Autodesk Fusion 360 part; units mm, degrees
sketch "Sketch1" plane through (0, 0, 0) normal (0, 0, 1) x (1, 0, 0)
  arc A0 (21.59, 0) -> (24.13, 2.54) centre (21.59, 2.54) ccw
  arc A1 (0, 2.54) -> (2.54, 0) centre (2.54, 2.54) ccw
  line L0 (21.59, 0) -> (2.54, 0)
  arc A2 (2.54, 15.24) -> (0, 12.7) centre (2.54, 12.7) ccw
  line L1 (24.13, 12.7) -> (24.13, 2.54)
  line L2 (0, 2.54) -> (0, 12.7)
  line L3 (2.54, 15.24) -> (21.59, 15.24)
  arc A3 (24.13, 12.7) -> (21.59, 15.24) centre (21.59, 12.7) ccw
  arc A4 (20.9931, 9.293) -> (19.9009, 9.293) centre (20.447, 9.293) ccw
  line L4 (2.159, 1.651) -> (3.937, 1.651)
  line L5 (3.937, 1.651) -> (3.937, 3.429)
  line L6 (2.159, 1.651) -> (3.937, 1.651)
  line L7 (3.937, 1.651) -> (3.937, 3.429)
  line L8 (3.937, 3.429) -> (2.159, 3.429)
  arc A5 (20.9931, 5.793) -> (19.9009, 5.793) centre (20.447, 5.793) ccw
  arc A6 (19.9009, 9.293) -> (20.9931, 9.293) centre (20.447, 9.293) ccw
  arc A7 (19.9009, 9.293) -> (20.9931, 9.293) centre (20.447, 9.293) ccw
  line L9 (2.159, 3.429) -> (2.159, 1.651)
  line L10 (2.159, 3.429) -> (2.159, 1.651)
  arc A8 (20.9931, 9.293) -> (19.9009, 9.293) centre (20.447, 9.293) ccw
  arc A9 (19.9009, 5.793) -> (20.9931, 5.793) centre (20.447, 5.793) ccw
  arc A10 (20.9931, 5.793) -> (19.9009, 5.793) centre (20.447, 5.793) ccw
  line L11 (3.937, 3.429) -> (2.159, 3.429)
  arc A11 (19.9009, 5.793) -> (20.9931, 5.793) centre (20.447, 5.793) ccw
  circle A12 centre (21.59, 2.286) radius 1.27
  circle A13 centre (21.59, 12.954) radius 1.27
  circle A14 centre (3.048, 2.54) radius 0.635
  circle A15 centre (3.048, 5.08) radius 0.635
  circle A16 centre (3.048, 7.62) radius 0.635
  circle A17 centre (3.048, 10.16) radius 0.635
  circle A18 centre (3.048, 12.7) radius 0.635
  circle A19 centre (3.048, 5.08) radius 1
  circle A20 centre (3.048, 7.62) radius 1
  circle A21 centre (3.048, 10.16) radius 1
  circle A22 centre (3.048, 12.7) radius 1
  dimension "d1" = 2.54
  dimension "d2" = 2.54
  dimension "d5" = 1.27
  dimension "d8" = 0
  dimension "d9" = 2.54
  dimension "d10" = 2
  dimension "d13" = 0
  dimension "d14" = 2.54
extrude "Extrude1" add sketch "Sketch1" along normal blind 1.6 contours A0 A1 L0 A2 L1 L2 L3 A3 | L4 L5 L6 L7 L8 L9 L10 L11 | A19 | A20 | A21 | A22
extrude "Extrude2" add sketch "Sketch1" along normal blind 0.2 from surface at 1.6 contours L4 L5 L6 L7 L8 L9 L10 L11 | A19 | A20 | A21 | A22
sketch "Sketch2" plane through (0, 0, 1.6) normal (0, 0, 1) x (-1, 0, 0)
  circle A0 centre (-3.048, -12.7) radius 1
  line L0 (-3.937, -1.651) -> (-2.159, -1.651)
  line L1 (-2.159, -1.651) -> (-2.159, -3.429)
  line L2 (-2.159, -3.429) -> (-3.937, -3.429)
  line L3 (-3.937, -3.429) -> (-3.937, -1.651)
  circle A1 centre (-3.048, -10.16) radius 1
  circle A2 centre (-3.048, -5.08) radius 1
  circle A3 centre (-3.048, -7.62) radius 1
  circle A4 centre (-21.59, -2.286) radius 1.27
  circle A5 centre (-20.447, -9.293) radius 0.5461
  circle A6 centre (-21.59, -12.954) radius 1.27
  circle A7 centre (-20.447, -5.793) radius 0.5461
  arc A8 (-21.59, 0) -> (-24.13, -2.54) centre (-21.59, -2.54) ccw
  line L4 (-24.13, -2.54) -> (-24.13, -12.7)
  arc A9 (-24.13, -12.7) -> (-21.59, -15.24) centre (-21.59, -12.7) ccw
  line L5 (-21.59, -15.24) -> (-2.54, -15.24)
  arc A10 (-2.54, -15.24) -> (0, -12.7) centre (-2.54, -12.7) ccw
  line L6 (0, -12.7) -> (0, -2.54)
  arc A11 (0, -2.54) -> (-2.54, 0) centre (-2.54, -2.54) ccw
  line L7 (-2.54, 0) -> (-21.59, 0)
  line L8 (-7.25, -3.5) -> (-5.75, -3.5)
  line L9 (-5.75, -3.5) -> (-5.75, -6.5)
  line L10 (-5.75, -6.5) -> (-7.25, -6.5)
  line L11 (-7.25, -6.5) -> (-7.25, -3.5)
  line L12 (-7.25, -3.5) -> (-5.75, -6.5) construction
  line L13 (-5.75, -3.5) -> (-7.25, -6.5) construction
  line L14 (-9.75, -2.5) -> (-8.25, -2.5)
  line L15 (-8.25, -2.5) -> (-8.25, -5.5)
  line L16 (-8.25, -5.5) -> (-9.75, -5.5)
  line L17 (-9.75, -5.5) -> (-9.75, -2.5)
  line L18 (-9.75, -2.5) -> (-8.25, -5.5) construction
  line L19 (-8.25, -2.5) -> (-9.75, -5.5) construction
  line L20 (-15, -3.5) -> (-11, -3.5)
  line L21 (-11, -3.5) -> (-11, -7.5)
  line L22 (-11, -7.5) -> (-15, -7.5)
  line L23 (-15, -7.5) -> (-15, -3.5)
  line L24 (-15, -3.5) -> (-11, -7.5) construction
  line L25 (-11, -3.5) -> (-15, -7.5) construction
  line L26 (-9, -9.25) -> (-6, -9.25)
  line L27 (-6, -9.25) -> (-6, -10.75)
  line L28 (-6, -10.75) -> (-9, -10.75)
  line L29 (-9, -10.75) -> (-9, -9.25)
  line L30 (-9, -9.25) -> (-6, -10.75) construction
  line L31 (-6, -9.25) -> (-9, -10.75) construction
  line L32 (-6.5, -7.25) -> (-9.5, -7.25)
  line L33 (-9.5, -7.25) -> (-9.5, -8.75)
  line L34 (-9.5, -8.75) -> (-6.5, -8.75)
  line L35 (-6.5, -8.75) -> (-6.5, -7.25)
  line L36 (-6.5, -7.25) -> (-9.5, -8.75) construction
  line L37 (-9.5, -7.25) -> (-6.5, -8.75) construction
  circle A12 centre (-8, -13) radius 1.25
  line L38 (-14, -12) -> (-11, -12)
  line L39 (-11, -12) -> (-11, -13.5)
  line L40 (-11, -13.5) -> (-14, -13.5)
  line L41 (-14, -13.5) -> (-14, -12)
  line L42 (-14, -12) -> (-11, -13.5) construction
  line L43 (-11, -12) -> (-14, -13.5) construction
  line L44 (-12, -8.5) -> (-10.5, -8.5)
  line L45 (-10.5, -8.5) -> (-10.5, -11.5)
  line L46 (-10.5, -11.5) -> (-12, -11.5)
  line L47 (-12, -11.5) -> (-12, -8.5)
  line L48 (-12, -8.5) -> (-10.5, -11.5) construction
  line L49 (-10.5, -8.5) -> (-12, -11.5) construction
  line L50 (-19, -2.5) -> (-16, -2.5)
  line L51 (-16, -2.5) -> (-16, -4)
  line L52 (-16, -4) -> (-19, -4)
  line L53 (-19, -4) -> (-19, -2.5)
  line L54 (-19, -2.5) -> (-16, -4) construction
  line L55 (-16, -2.5) -> (-19, -4) construction
  line L56 (-19, -6) -> (-19, -4.5)
  line L57 (-19, -4.5) -> (-16, -4.5)
  line L58 (-16, -4.5) -> (-16, -6)
  line L59 (-16, -6) -> (-19, -6)
  line L60 (-19, -8) -> (-19, -6.5)
  line L61 (-19, -6.5) -> (-16, -6.5)
  line L62 (-16, -6.5) -> (-16, -8)
  line L63 (-16, -8) -> (-19, -8)
  line L64 (-19, -10) -> (-19, -8.5)
  line L65 (-19, -8.5) -> (-16, -8.5)
  line L66 (-16, -8.5) -> (-16, -10)
  line L67 (-16, -10) -> (-19, -10)
  line L68 (-6.5, -11.5) -> (-9.5, -11.5)
  line L69 (-9.5, -11.5) -> (-9.5, -14.5)
  line L70 (-9.5, -14.5) -> (-6.5, -14.5)
  line L71 (-6.5, -14.5) -> (-6.5, -11.5)
  line L72 (-6.5, -11.5) -> (-9.5, -14.5) construction
  line L73 (-9.5, -11.5) -> (-6.5, -14.5) construction
  point P0 (-6.5, -5)
  point P1 (-9, -4)
  point P2 (-13, -5.5)
  point P3 (-7.5, -10)
  point P4 (-8, -8)
  point P5 (-12.5, -12.75)
  point P6 (-11.25, -10)
  point P7 (-17.5, -3.25)
  point P8 (-8, -13)
  dimension "d18" = 1.5
  dimension "d19" = 3
  dimension "d20" = 1.5
  dimension "d21" = 3
  dimension "d22" = 4
  dimension "d23" = 4
  dimension "d24" = 3
  dimension "d25" = 1.5
  dimension "d26" = 3
  dimension "d27" = 1.5
  dimension "d28" = 2.5
  dimension "d29" = 1.5
  dimension "d30" = 3
  dimension "d31" = 3
  dimension "d32" = 1.5
  dimension "d33" = 3
  dimension "d34" = 1.5
  dimension "d37" = 0
  dimension "d38" = -2
  dimension "d43" = 3
  dimension "d44" = 3
extrude "Extrude3" add sketch "Sketch2" along normal blind 0.5 contours L8 L9 L10 L11 | L32 L33 L34 L35 | L44 L45 L46 L47
extrude "Extrude4" add sketch "Sketch2" along normal blind 1 contours L14 L15 L16 L17 | L20 L21 L22 L23 | L26 L27 L28 L29 | L38 L39 L40 L41 | L50 L51 L52 L53 | L56 L57 L58 L59 | L60 L61 L62 L63 | L64 L65 L66 L67
extrude "Extrude5" add sketch "Sketch2" along normal blind 1 contours A12 | L68 L69 L70 L71
extrude "Extrude6" add sketch "Sketch2" along normal blind 0.5 from surface at 1 contours A12
Input: part model. Units: mm. Frame: model coordinates. A direction names the side the tool comes from. Give positions to 0.01 mm unless a question says otherwise; leave off trailing zeros. Order: outer loops, then holes, each group sorted by start corner. A loop starts at its lowest first (then second) coordinate and runs counter-clockwise, first axis right, second up. Notation, with made-up numbers: (25.5, -8) - (52.5, -8) arc R26 cw to (52.5, 18) - close; hole circle Ø9 at (-18.75, 45.25). An arc over 180 degrees is marked (long way). Use a Markdown table: item, result.
(1) Section query B-B (x = 8). Output: boundary loops of the cut face in (y, z), then the cut area to 3 significant figures.
Computed values:
| item | result |
|---|---|
| outline | (0, 0) - (15.24, 0) - (15.24, 1.6) - (14.5, 1.6) - (14.5, 2.6) - (14.25, 2.6) - (14.25, 3.1) - (11.75, 3.1) - (11.75, 2.6) - (11.5, 2.6) - (11.5, 1.6) - (10.75, 1.6) - (10.75, 2.6) - (9.25, 2.6) - (9.25, 1.6) - (8.75, 1.6) - (8.75, 2.1) - (7.25, 2.1) - (7.25, 1.6) - (0, 1.6) - close |
| area | 30.9 mm2 |
(2) Section query A-A (y = 10.5). Output: boundary loops of the cut face in (x, z), then the cut area to 3 significant figures.
Computed values:
| item | result |
|---|---|
| outline | (0, 0) - (2.51, 0) - (2.51, 1.8) - (2.11, 1.8) - (2.11, 1.6) - (0, 1.6) - close; (3.58, 0) - (24.13, 0) - (24.13, 1.6) - (12, 1.6) - (12, 2.1) - (10.5, 2.1) - (10.5, 1.6) - (9, 1.6) - (9, 2.6) - (6, 2.6) - (6, 1.6) - (3.99, 1.6) - (3.99, 1.8) - (3.58, 1.8) - close |
| area | 40.8 mm2 |
(3) Access query for faces 1 (the flat face through (16, 7, 2)), 2 (the flat face through (17, 10, 2)), 3 (the flat face through (8, 11.5, 2)), 4 (the flat face through (13, 7.5, 2)). Directions: +Z, -Z, +X, -X, +Y, -Y. A direction counts if a zero-diameter tool reaches every point of the face in a straight line with its end or side. Return the directions, or none.
Computed values:
| item | result |
|---|---|
| face 1 | +Z, +Y, -Y |
| face 2 | +Z, +X, +Y |
| face 3 | +Z, -X |
| face 4 | +Z |
(4) Pin query (flat end, axial travel): pin 1 (0.5 mm diameter, centred on y = 9, z = 2, fed in from +X); pin 2 (1.6 mm diameter, centred on x = 7, y = 5, fed in from +Z); pin 3 (2 mm diameter, centred on x = 21.59, y = 2.286, fed in from +Z); pin 4 (0.5 mm diameter, centred on x = 17.5, z = 2, fed in from +Y). Return the tip coordinate at first contact, or that it passes through.
Computed values:
| item | result |
|---|---|
| pin 1 | stops at x = 19 |
| pin 2 | stops at z = 2.1 |
| pin 3 | passes through |
| pin 4 | stops at y = 10 |
(5) Section query D-D (x = 11.5). Output: boundary loops of the cut face in (y, z).
Computed values:
| item | result |
|---|---|
| outline | (0, 0) - (15.24, 0) - (15.24, 1.6) - (13.5, 1.6) - (13.5, 2.6) - (12, 2.6) - (12, 1.6) - (11.5, 1.6) - (11.5, 2.1) - (8.5, 2.1) - (8.5, 1.6) - (7.5, 1.6) - (7.5, 2.6) - (3.5, 2.6) - (3.5, 1.6) - (0, 1.6) - close |
(6) Section query C-C (z = 0.3). State how many separate pieces and enclosed holes the cut face has, then the cut area to 3 significant figures.
Computed values:
| item | result |
|---|---|
| separate pieces | 1 |
| enclosed holes | 9 |
| area | 344 mm2 |
(7) Line query: line 1 (X direction, y = 12.75, z = 1.7); line 2 (Y direction, x = 21.59, z = 0.6); line 3 (Y direction, x = 17.75, z = 2.4). Output: solid intervals per line, ascending. Write a range as from..to.
Computed values:
| item | result |
|---|---|
| line 1 | x = 2.05..2.41, 3.68..4.05, 6.5..9.5, 11..14 |
| line 2 | y = 0..1.02, 3.56..11.68, 14.22..15.24 |
| line 3 | y = 2.5..4, 4.5..6, 6.5..8, 8.5..10 |
